Build history of the part. All positions in model axes, mm. A direction names the side the tool comes from. Round coordinates to 2 decimals unless told otherwise and drop trailing zeros. Write each loop counter-clockwise with the first axis right and the second up, starting at its lowest first coordinate (ties: lowest second). Pieces come first, ordered by that corner, then holes. Notation, with made-up numbers: M 13.25,76.5 L 29.25,76.5 A23 ccw 29.25,98.5 Z; hole C -32,78 d11. An arc over 180 degrees is marked long. Write item = value, one per line.
from build123d import *

# Parameters (mm, degrees)
CROQUIS1_R              = 9.75
SALIENTE_EXTRUIR1_DEPTH = 6


with BuildPart() as part:
    # Croquis1 → Saliente-Extruir1 (new body)
    with BuildSketch(Plane.XY):
        with BuildLine():
            Line((-12.5, 0), (-12.5, -10))
            Line((-12.5, -10), (-7.5, -10))
            Line((-7.5, -10), (-7.5, -15))
            Line((-7.5, -15), (4.5, -15))
            Line((4.5, -15), (4.5, -10))
            Line((4.5, -10), (16.5, -10))
            Line((16.5, -10), (16.5, -15))
            Line((16.5, -15), (28.5, -15))
            Line((28.5, -15), (28.5, -10))
            Line((28.5, -10), (33.5, -10))
            Line((33.5, -10), (24.60996669, 24.748813068))
            ThreePointArc((24.60996669, 24.748813068), (10.938683829, 34.052743456), (0, 21.650635095))
            Line((0, 21.650635095), (0, 20.155644371))
            ThreePointArc((0, 20.155644371), (-1.501634144, 14.885181604), (-5.555555556, 11.197580206))
            ThreePointArc((-5.555555556, 11.197580206), (-10.62295732, 6.588078459), (-12.5, 0))
        make_face()
        Circle(CROQUIS1_R, mode=Mode.SUBTRACT)
        with Locations((12.5, 21.650635095)):
            Circle(CROQUIS1_R, mode=Mode.SUBTRACT)
    extrude(amount=SALIENTE_EXTRUIR1_DEPTH)


solid = part.part
1. Band-saw the part on B-B (x = 12.5). List the corners of the cut face in (y, z).
Responses:
outline = M -10,0 L 11.9,0 L 11.9,6 L -10,6 Z; M 31.4,0 L 34.15,0 L 34.15,6 L 31.4,6 Z
2. Probe probe 1 along Y at (x, z) = (12.5, 0.65); probe 2 along Y at (x, z) = (-6, 4.15); probe 3 along X at (y, z) = (2, 3). List the from-to ranges inside material, lowest first.
Responses:
probe_1 = -10 to 11.9, 31.4 to 34.15
probe_2 = -15 to -7.69, 7.69 to 10.97
probe_3 = -12.34 to -9.54, 9.54 to 30.43
3. Tool access for faces 5 (the face through (-7.5, -12, 3)), 6 (the face through (0, 21, 3)), 7 (the face through (31, -10, 3)), 8 (the face through (15, 4, 0)), 9 (the face through (16.5, -12, 3)): list every direction of +Z, -Z, +X, -X, +Y, -Y with a clear straight run to the whole face (end or side of a thin tool).
Responses:
face_5 = +Z, -Z, -X, -Y
face_6 = +Z, -Z, -X, +Y
face_7 = +Z, -Z, +X, -Y
face_8 = -Z, +X, -X, +Y, -Y
face_9 = +Z, -Z, -Y
4. Band-saw the part on A-A (z = 2.05). List the corners of the cut face in (x, y), plus the area to 3 significant figures.
Responses:
outline = M -12.5,-10 L -7.5,-10 L -7.5,-15 L 4.5,-15 L 4.5,-10 L 16.5,-10 L 16.5,-15 L 28.5,-15 L 28.5,-10 L 33.5,-10 L 24.61,24.75 A12.5 ccw 0,21.65 L 0,20.16 A10 cw -5.56,11.2 A12.5 ccw -12.5,0 Z; hole C 0,0 d19.5; hole C 12.5,21.65 d19.5
area = 958 mm²
5. Band-saw the part on D-D (x = 27.5). List the corners of the cut face in (y, z), plus the area to 3 significant figures.
Responses:
outline = M -15,0 L 13.45,0 L 13.45,6 L -15,6 Z
area = 171 mm²
6. Band-saw the part on C-C (y = 13). List the corners of the cut face in (x, z), plus the area to 3 significant figures.
Responses:
outline = M -3.01,0 L 8,0 L 8,6 L -3.01,6 Z; M 17,0 L 27.62,0 L 27.62,6 L 17,6 Z
area = 130 mm²
7. Flat gauge pins, fed straight in: pin 1 (2.5 mm diameter, centred on y = -11.5, z = 3, fed in from +X); pin 2 (2 mm diameter, centred on y = 18.5, z = 1, fed in from -X); pin 3 (2.5 mm diameter, centred on y = -13.5, z = 3, fed in from -X); pin 4 (5 mm diameter, centred on x = -4.5, y = 13, fed in from +Z). Where does each tip first touch, or does it go through?
Responses:
pin_1 = 28.5
pin_2 = -0.36
pin_3 = -7.5
pin_4 = 6
8. Mould opens along Y. For faces 1 (the face through (29.117, 7.131, 2.958)), 2 (the face through (-10, -10, 3)), 3 (the face through (4.5, -13, 3)), 4 (the face through (11.231, 31.318, 2.958)) say: pulls with the +Y half, pulls with the -Y half, needs draft (parallel to the pull), parting line crosses it, or undercut.
Responses:
face_1 = pulls with the +Y half
face_2 = pulls with the -Y half
face_3 = needs draft
face_4 = undercut
